Read the model definition and answer for the solid it produces. Units are mm, in the model's axes. Face numbers are marked on the shaded views. A direction names the side the tool comes from. Give positions to 0.01 mm unless a question says otherwise; leave off trailing zeros. Write each loop counter-clockwise with the first axis right and the second up, starting at its lowest first coordinate (ties: lowest second). Pieces come first, ordered by that corner, then holes. Notation, with made-up numbers: (35.5, -35) -> (45.5, -35) arc R10 cw to (45.5, -31) -> close; hole circle Ø9 at (1.5, -33). An arc over 180 degrees is marked (long way). Answer as CSV lines item,"result". Start each with the question number.
1. The part is cut by section C-C, the plane y = 52.5. Determine the outline of the cut face in (x, z), and give its area (3 significant figures).
2. The part is cut by section A-A, the plane x = 0. Determine the outline of the cut face in (y, z), and give its area (3 significant figures).
3. Given pin 1 (2.5 mm diameter, centred on y = 12.5, z = 27, fed in from -X); pin 2 (12 mm diameter, centred on x = 24.5, y = 28, fed in from -Z); pin 3 (12 mm diameter, centred on x = 33, z = 11.5, fed in from -Y); pin 4 (8 mm diameter, centred on x = -18, z = 7, fed in from +Y), each flat-ended and moving along its own axis, determine where each tip first touches the part or whether it passes through.
4. For a pull along X with two mould halves and no side action, classify the marked faces 1, 2 and 3 as pulls with the +X half, pulls with the -X half, needs draft (parallel to the pull), parting line crosses it, or undercut.
5. The part is cut by section D-D, the plane y = 20. Determine the outline of the cut face in (x, z), and give its area (3 significant figures).
6. A tool of negligible diameter and unlimited length cuts with its end or side. For the marked faces 4, 5, 6 and 7, from which of +Z, -Z, +X, -X, +Y, -Y can it reach the whole face along a straight path? Write none if from no direction.
7. Find the intervals of material crossed by line 1 (Z direction, x = 0, y = 27.05); line 2 (Y direction, x = -23.5, z = 45.5); line 3 (Y direction, x = -27, z = 42), in increasing order.
8. The part is cut by section B-B, the plane z = 35. Give the number of separate pieces and of enclosed holes in the cut face, and give its area (3 significant figures).
from build123d import *

# Parameters (mm, degrees)
SCHIZZO1_W                   = 20
SCHIZZO1_H                   = 20
ESTRUSIONE_ESTRUSIONE1_DEPTH = 60
RACCORDO1_R                  = 20
SCHIZZO8_R                   = 2.5
TAGLIO_ESTRUSIONE3_DEPTH     = 5
TAGLIO_ESTRUSIONE4_DEPTH     = 113.253811369
RACCORDO2_R                  = 10
RACCORDO3_R                  = 4
SCHIZZO11_R                  = 2.5
TAGLIO_ESTRUSIONE5_DEPTH     = 113.253811369


with BuildPart() as part:
    # Schizzo1 → Estrusione-Estrusione1 (new body)
    with BuildSketch(Plane.XY):
        Polygon((25, 0), (-25, 0), (-35.103629711, 17.5), (-17.783121635, 27.5), (-47.783121635, 79.461524227), (-43.452994616, 81.961524227), (-13.452994616, 30), (13.452994616, 30), (43.452994616, 81.961524227), (47.783121635, 79.461524227), (17.783121635, 27.5), (35.103629711, 17.5), align=None)
        with Locations((0, 15)):
            Rectangle(SCHIZZO1_W, SCHIZZO1_H, mode=Mode.SUBTRACT)
    extrude(amount=ESTRUSIONE_ESTRUSIONE1_DEPTH)

    # Raccordo1
    raccordo1_edges = [part.edges().sort_by_distance(p)[0] for p in [
        (25, 0, 30),
        (-25, 0, 30),
    ]]
    fillet(raccordo1_edges, radius=RACCORDO1_R)

    # Schizzo8 → Taglio-Estrusione3 (cut)
    with BuildSketch(Plane(origin=(-1.429491924, -0.825317547, 0), x_dir=(0, 0, 1), z_dir=(-0.8660254037844398, -0.49999999999999806, 0))):
        with Locations(Location((10, 47.707259422, 0), (0, 0, 270))):
            Circle(SCHIZZO8_R)
        with Locations(Location((50, 47.707259422, 0), (0, 0, 90))):
            Circle(SCHIZZO8_R)
        with BuildLine():
            Line((12.5, 85.707259422), (12.5, 75.707259422))
            ThreePointArc((12.5, 75.707259422), (10, 73.207259422), (7.5, 75.707259422))
            Line((7.5, 75.707259422), (7.5, 85.707259422))
            ThreePointArc((7.5, 85.707259422), (10, 88.207259422), (12.5, 85.707259422))
        make_face()
        with BuildLine():
            Line((47.5, 85.707259422), (47.5, 75.707259422))
            ThreePointArc((47.5, 75.707259422), (50, 73.207259422), (52.5, 75.707259422))
            Line((52.5, 75.707259422), (52.5, 85.707259422))
            ThreePointArc((52.5, 85.707259422), (50, 88.207259422), (47.5, 85.707259422))
        make_face()
    taglio_estrusione3 = extrude(amount=-TAGLIO_ESTRUSIONE3_DEPTH, mode=Mode.SUBTRACT)

    # Specchia1: Taglio-Estrusione3 across plane
    add(taglio_estrusione3.mirror(Plane(origin=(0, 0, 0), x_dir=(0, 0, 1), z_dir=(1, 0, 0))), mode=Mode.SUBTRACT)

    # Schizzo10 → Taglio-Estrusione4 (cut, through all)
    with BuildSketch(Plane(origin=(0, 0, 0), x_dir=(-1, 0, 0), z_dir=(0, 0, -1))):
        with BuildLine():
            Line((-28.773502692, 16.535898385), (-13.452994616, 25.381197846))
            Line((-13.452994616, 25.381197846), (-13.452994616, 5))
            ThreePointArc((-13.452994616, 5), (-20.952994616, 7.009618943), (-26.443375673, 12.5))
            Line((-26.443375673, 12.5), (-28.773502692, 16.535898385))
        make_face()
        with BuildLine():
            Line((13.452994616, 25.381197846), (13.452994616, 5))
            ThreePointArc((13.452994616, 5), (20.952994616, 7.009618943), (26.443375673, 12.5))
            Line((26.443375673, 12.5), (28.773502692, 16.535898385))
            Line((28.773502692, 16.535898385), (13.452994616, 25.381197846))
        make_face()
    extrude(amount=-TAGLIO_ESTRUSIONE4_DEPTH, mode=Mode.SUBTRACT)

    # Raccordo2
    raccordo2_edges = [part.edges().sort_by_distance(p)[0] for p in [
        (-13.452994616, 30, 30),
        (13.452994616, 30, 30),
    ]]
    fillet(raccordo2_edges, radius=RACCORDO2_R)

    # Raccordo3
    raccordo3_edges = [part.edges().sort_by_distance(p)[0] for p in [
        (28.773502692, 16.535898385, 30),
        (13.452994616, 25.381197846, 30),
        (13.452994616, 5, 30),
        (-13.452994616, 5, 30),
        (-13.452994616, 25.381197846, 30),
        (-28.773502692, 16.535898385, 30),
    ]]
    fillet(raccordo3_edges, radius=RACCORDO3_R)

    # Schizzo11 → Taglio-Estrusione5 (cut, through all)
    with BuildSketch(Plane.XZ):
        with Locations((0, 48)):
            Circle(SCHIZZO11_R)
        with Locations((0, 12)):
            Circle(SCHIZZO11_R)
    extrude(amount=-TAGLIO_ESTRUSIONE5_DEPTH, mode=Mode.SUBTRACT)


solid = part.part
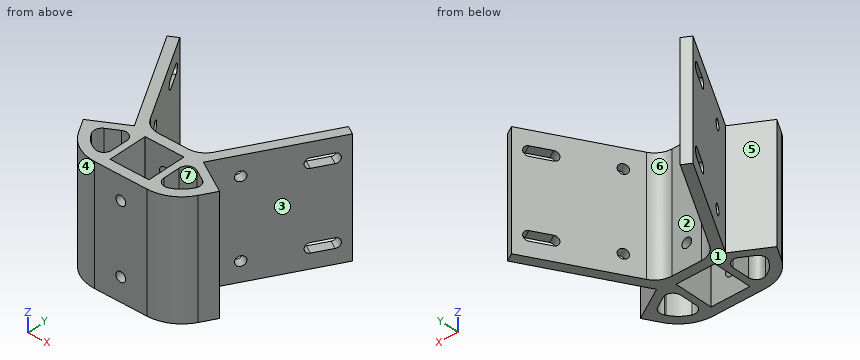
Results found:
1,outline,"(-32.22, 0) -> (-26.44, 0) -> (-26.44, 60) -> (-32.22, 60) -> close; (26.44, 0) -> (32.22, 0) -> (32.22, 60) -> (26.44, 60) -> close"
1,area,"693 mm²"
2,outline,"(0, 0) -> (5, 0) -> (5, 9.5) -> (0, 9.5) -> close; (0, 14.5) -> (5, 14.5) -> (5, 45.5) -> (0, 45.5) -> close; (0, 50.5) -> (5, 50.5) -> (5, 60) -> (0, 60) -> close; (25, 0) -> (30, 0) -> (30, 9.5) -> (25, 9.5) -> close; (25, 14.5) -> (30, 14.5) -> (30, 45.5) -> (25, 45.5) -> close; (25, 50.5) -> (30, 50.5) -> (30, 60) -> (25, 60) -> close"
2,area,"500 mm²"
3,pin 1,"stops at x = -32.94"
3,pin 2,"stops at z = 0"
3,pin 3,"stops at y = 5.29"
3,pin 4,"stops at y = 44.8"
4,face 1,"needs draft"
4,face 2,"undercut"
4,face 3,"pulls with the +X half"
5,outline,"(-30.77, 0) -> (-22.77, 0) -> (-22.77, 60) -> (-30.77, 60) -> close; (-13.76, 0) -> (-10, 0) -> (-10, 60) -> (-13.76, 60) -> close; (10, 0) -> (13.76, 0) -> (13.76, 60) -> (10, 60) -> close; (22.77, 0) -> (30.77, 0) -> (30.77, 60) -> (22.77, 60) -> close"
5,area,"1,410 mm²"
6,face 4,"+Z, -Z, -X, -Y"
6,face 5,"+Z, -Z, -X"
6,face 6,"+Z, -Z, +Y"
6,face 7,"+Z, -Z"
7,line 1,"z = 0 to 9.5, 14.5 to 45.5, 50.5 to 60"
7,line 2,"y = 2.71 to 8.86, 19.58 to 24.2, 37.4 to 47.4"
7,line 3,"y = 5.29 to 13.53, 16.61 to 22.18, 43.46 to 53.46"
8,separate pieces,"1"
8,enclosed holes,"3"
8,area,"1,480 mm²"
